The model under review builds one solid part; all positions refer to its coordinate system, in mm. A direction names the side the tool comes from. Round coordinates to 2 decimals unless told otherwise and drop trailing zeros. Order: outer loops, then holes, each group sorted by start corner. A loop starts at its lowest first (then second) coordinate and runs counter-clockwise, first axis right, second up. Notation, with made-up numbers: M -36.5,-25 L -4.5,-25 A20 ccw -4.5,-9 Z; hole C 19.25,10 d6. An arc over 180 degrees is marked long. Answer as a JSON object with one key per item and string values. Group by question number.
1. Add section A-A on y = -2.5. State the section outline as (x, z) points.
2. Add section B-B on y = -9.75. State the section outline as (x, z) points.
3. To check wall thickness, follow probe 1 along Z at (x, y) = (-1.75, -0.75); probe 2 along Z at (x, y) = (1, -1.75); probe 3 along X at (y, z) = (-0.75, 2.75). State the ranges of each line that lie inside material, in increasing order. Write a range as [from, to].
4. Clearance check with flat-ended pins moving along their axes: P1, Ø1.2, axis at y = -0.5, z = 2, coming from the +X side; P2, Ø0.5, axis at y = -0.5, z = 2, coming from the -X side; P3, Ø0.6, axis at y = -0.5, z = 0, coming from the +X side; P4, Ø4, axis at y = -10.5, z = -1.5, coming from the -X side. State where each tip first meets the part, or that it passes through.
5. Machinability: for faces 1 (the face through (-1.52, -6.29, 1.66)), 2 (the face through (1, 0, -1)), 3 (the face through (-0.5, -0.7, -1.6)), which of the approach directions +Z, -Z, +X, -X, +Y, -Y give a long, thin tool a straight path to every point of the face, cutting with its end or side? Answer none if there is none.
6. Mouldability with a two-part tool opening along Z and no side actions: class faces 4 (the face through (3.905, -0.222, 0.867)), 5 (the face through (-1.6, -0.7, -0.5)), 6 (the face through (0, -12, 0)) as released by +Z, released by -Z, zero draft, split by the parting line, or undercut.
```python
from build123d import *

# Parameters (mm, degrees)
CUT_EXTRUDE2_REACH = 15.266
CHAMFER1_SIZE      = 0.5
FILLET1_R          = 0.4


with BuildPart() as part:
    # Sketch1 → Revolve1 (revolve)
    with BuildSketch(Plane.XY, mode=Mode.PRIVATE) as revolve1_sk:
        Polygon((0, 0), (0, -12), (2.25, -12), (2.25, -2.2), (4, -0.45), (4, 0), align=None)
    revolve(revolve1_sk.sketch.rotate(Axis((0, 0, 0), (0, 1, 0)), 90), axis=Axis((0, 0, 0), (0, 1, 0)))

    # Sketch4 → Cut-Revolve1 (revolve, cut)
    with BuildSketch(Plane(origin=(0, 0, 0), x_dir=(0, 0, -1), z_dir=(1, 0, 0))):
        Polygon((1.85, -12), (2.25, -10.5), (2.25, -12), align=None)
    revolve(axis=Axis((0, 0, 0), (0, -1, 0)), mode=Mode.SUBTRACT)

    # Cut-Extrude2: up to this cone (the profile starts inside it)
    cut_extrude2_end = Plane(origin=(0, 0, 0), z_dir=(0, 1, 0)).offset(-3.035785438) * Cone(1e-06, 21.837572875, 21.837571875, align=(Align.CENTER, Align.CENTER, Align.MIN), mode=Mode.PRIVATE)
    # Sketch6 → Cut-Extrude2 (cut, up to the surface)
    with BuildSketch(Plane(origin=(0, 0, 0), x_dir=(1, 0, 0), z_dir=(0, 1, 0)), mode=Mode.PRIVATE) as cut_extrude2_sk1:
        Polygon((-0.5, 2.25), (0.5, 2.25), (0.5, 0.5), (2.25, 0.5), (2.25, -0.5), (0.5, -0.5), (0.5, -2.25), (-0.5, -2.25), (-0.5, -0.5), (-2.25, -0.5), (-2.25, 0.5), (-0.5, 0.5), align=None)
    cut_extrude2_tool1 = extrude(cut_extrude2_sk1.sketch, amount=-CUT_EXTRUDE2_REACH, mode=Mode.PRIVATE) & cut_extrude2_end
    add(cut_extrude2_tool1.solids().sort_by_distance((0, 0, 0))[0], mode=Mode.SUBTRACT)

    # Chamfer1
    chamfer1_edges = [part.edges().sort_by_distance(p)[0] for p in [
        (0.5, -1.164339828, 0.5),
        (-0.5, -1.164339828, 0.5),
        (0.5, -1.164339828, -0.5),
        (-0.5, -1.164339828, -0.5),
    ]]
    chamfer(chamfer1_edges, length=CHAMFER1_SIZE)

    # Fillet1
    fillet1_edges = [part.edges().sort_by_distance(p)[0] for p in [
        (-1, -0.958876224, 0.5),
        (-0.5, -0.958876224, 1),
        (0.5, -0.958876224, 1),
        (1, -0.958876224, 0.5),
        (1, -0.958876224, -0.5),
        (0.5, -0.958876224, -1),
        (-0.5, -0.958876224, -1),
        (-1, -0.958876224, -0.5),
    ]]
    fillet(fillet1_edges, radius=FILLET1_R)


solid = part.part
```
Recorded:
{
 "1": {"outline": "C 0,0 d4.5; hole C 0,0 d1.07"},
 "2": {"outline": "C 0,0 d4.5"},
 "3": {"probe 1": "z = [-3.26, -0.5], [0.5, 3.26]", "probe 2": "z = [-2.51, -0.54], [0.54, 2.51]", "probe 3": "x = [-2.48, 2.48]"},
 "4": {"P1": "stops at x = 3.75", "P2": "stops at x = -3.59", "P3": "stops at x = 4", "P4": "stops at x = -2.25"},
 "5": {"face 1": "-Y", "face 2": "+Z, -Z, +X, -X, +Y", "face 3": "+Y"},
 "6": {"face 4": "split by the parting line", "face 5": "undercut", "face 6": "zero draft"}
}
